```python
from build123d import *

# Parameters (mm, degrees)
SKETCH1_W           = 100
SKETCH1_H           = 50
SKETCH1_R           = 2.5
BOSS_EXTRUDE1_DEPTH = 10
SKETCH2_W           = 60
SKETCH2_H           = 60
BOSS_EXTRUDE2_DEPTH = 50
SKETCH3_R           = 15
CUT_EXTRUDE1_DEPTH  = 101
SKETCH5_R           = 2.5
CUT_EXTRUDE3_DEPTH  = 10


with BuildPart() as part:
    # Sketch1 → Boss-Extrude1 (new body)
    with BuildSketch(Plane.XY):
        Rectangle(SKETCH1_W, SKETCH1_H)
        with Locations((-42.5, 17.5)):
            Circle(SKETCH1_R, mode=Mode.SUBTRACT)
        with Locations((42.5, 17.5)):
            Circle(SKETCH1_R, mode=Mode.SUBTRACT)
        with Locations((42.5, -17.5)):
            Circle(SKETCH1_R, mode=Mode.SUBTRACT)
        with Locations((-42.5, -17.5)):
            Circle(SKETCH1_R, mode=Mode.SUBTRACT)
    extrude(amount=BOSS_EXTRUDE1_DEPTH)

    # Sketch2 → Boss-Extrude2 (add)
    with BuildSketch(Plane.XY.offset(10)):
        Rectangle(SKETCH2_W, SKETCH2_H)
    extrude(amount=BOSS_EXTRUDE2_DEPTH)

    # Sketch3 → Cut-Extrude1 (cut)
    with BuildSketch(Plane.ZY.offset(30)):
        with Locations((35, 0)):
            Circle(SKETCH3_R)
    extrude(amount=-CUT_EXTRUDE1_DEPTH, mode=Mode.SUBTRACT)

    # Sketch5 → Cut-Extrude3 (cut)
    with BuildSketch(Plane.XY.offset(60)):
        with Locations((-17.5, 17.5)):
            Circle(SKETCH5_R)
        with Locations((-2.5, 17.5)):
            Circle(SKETCH5_R)
        with Locations((-2.5, -17.5)):
            Circle(SKETCH5_R)
        with Locations((-17.5, -17.5)):
            Circle(SKETCH5_R)
    extrude(amount=-CUT_EXTRUDE3_DEPTH, mode=Mode.SUBTRACT)


solid = part.part
```
Geometry: final body of the model. Coordinates: model frame, mm. A direction names the side the tool comes from. Coordinates: 2 decimals unless noted, no trailing zeros. Write each loop counter-clockwise with the first axis right and the second up, starting at its lowest first coordinate (ties: lowest second). Pieces come first, ordered by that corner, then holes. Notation, with made-up numbers: M -31.75,9.25 L 18.25,9.25 A21 ccw 18.25,46.25 Z; hole C -16.5,-20 d10. An arc over 180 degrees is marked long. Answer as CSV lines item,"result". Start each with the question number.
Q1. Cut plane D-D on y = 17.5. Return the cut outline in (x, z), then the cut area to 3 significant figures.
Q2. Mould query, pull axis Y, two halves, no side actions, for faces 4 (the flat face through (-1, -25, 5)), 5 (the flat face through (-18, -17, 50)), 6 (the flat face through (0, -27, 10)). Classes: released by +Y, released by -Y, zero draft, split by the parting line, or undercut.
Q3. Cut plane B-B on y = 0. Return the cut outline in (x, z).
Q4. Cut plane A-A on x = -42.5. Return the cut outline in (y, z), then the cut area to 3 significant figures.
Q5. Pin query (flat end, axial travel): P1, Ø22, axis at x = 41.5, y = 8.5, coming from the +Z side; P2, Ø8, axis at x = -3.5, z = 3, coming from the +Y side; P3, Ø4, axis at x = -33, z = 36, coming from the +Y side; P4, Ø5.5, axis at x = -14, y = -28, coming from the -Z side. Return the tip coordinate at first contact, or that it passes through.
Q6. Cut plane C-C on z = 35. Return the cut outline in (x, y).
Q7. Reachability of faces 1 (the flat face through (0, 28, 10)), 2 (the flat face through (-30, 0, 18)), 3 (the cylindrical face through (-20, 17.6, 55.1)) from +Z, -Z, +X, -X, +Y, -Y: full face, straight path, thin tool, end or side. Return the list, or none.
Q8. Line query: line 1 (Y direction, x = 42.5, z = 6.25); line 2 (Y direction, x = -42, z = 5); line 3 (Y direction, x = 16.5, z = 35). Output: solid intervals per line, ascending. Write a range as from..to.
Findings below:
1,outline,"M -50,0 L -45,0 L -45,10 L -50,10 Z; M -40,0 L 40,0 L 40,10 L 30,10 L 30,60 L 0,60 L 0,50 L -5,50 L -5,60 L -15,60 L -15,50 L -20,50 L -20,60 L -30,60 L -30,10 L -40,10 Z; M 45,0 L 50,0 L 50,10 L 45,10 Z"
1,area,"3,800 mm2"
2,face 4,"released by -Y"
2,face 5,"undercut"
2,face 6,"zero draft"
3,outline,"M -50,0 L 50,0 L 50,10 L 30,10 L 30,20 L -30,20 L -30,10 L -50,10 Z; M -30,50 L 30,50 L 30,60 L -30,60 Z"
4,outline,"M -25,0 L -20,0 L -20,10 L -25,10 Z; M -15,0 L 15,0 L 15,10 L -15,10 Z; M 20,0 L 25,0 L 25,10 L 20,10 Z"
4,area,"400 mm2"
5,P1,"stops at z = 10"
5,P2,"stops at y = 25"
5,P3,"passes through"
5,P4,"stops at z = 10"
6,outline,"M -30,-30 L 30,-30 L 30,-15 L -30,-15 Z; M -30,15 L 30,15 L 30,30 L -30,30 Z"
7,face 1,"-Z, +X, -X, +Y"
7,face 2,"+Z, -X, +Y, -Y"
7,face 3,"+Z"
8,line 1,"y = -25..-20, -15..15, 20..25"
8,line 2,"y = -25..-19.95, -15.05..15.05, 19.95..25"
8,line 3,"y = -30..-15, 15..30"
